```python
from build123d import *

# Parameters (mm, degrees)
F2_DEPTH = 18
F3_DEPTH = 188


with BuildPart() as f2:
    # F0 (on Front) → F2 (new body)
    with BuildSketch(Plane.XZ):
        with BuildLine():
            Line((63.480214, -200), (80, -200))
            ThreePointArc((80, -200), (94.142136, -194.142136), (100, -180))
            Line((100, -180), (100, 200))
            Line((100, 200), (45, 200))
            Line((45, 200), (45, 218))
            Line((45, 218), (-45, 218))
            Line((-45, 218), (-45, 200))
            Line((-45, 200), (-100, 200))
            Line((-100, 200), (-100, -180))
            ThreePointArc((-100, -180), (-94.142136, -194.142136), (-80, -200))
            Line((-80, -200), (-63.480214, -200))
            ThreePointArc((-63.480214, -200), (-49.338079, -194.142136), (-43.480214, -180))
            Line((-43.480214, -180), (-43.480214, -110))
            Line((-43.480214, -110), (-43.480214, 90))
            ThreePointArc((-43.480214, 90), (-37.62235, 104.142136), (-23.480214, 110))
            Line((-23.480214, 110), (23.480214, 110))
            ThreePointArc((23.480214, 110), (37.62235, 104.142136), (43.480214, 90))
            Line((43.480214, 90), (43.480214, -110))
            Line((43.480214, -110), (43.480214, -180))
            ThreePointArc((43.480214, -180), (49.338079, -194.142136), (63.480214, -200))
        make_face()
    extrude(amount=F2_DEPTH)

    # F1 (on face) → F3 (cut)
    with BuildSketch(Plane.XZ):
        Polygon((9, 170.049076), (-9, 170.049076), (-9, 110.049076), (0, 110.049076), (9, 110.049076), align=None)
        Polygon((0, 110.049076), (-9, 110.049076), (-9, 70.049076), (9, 70.049076), (9, 110.049076), align=None)
    extrude(amount=F3_DEPTH, mode=Mode.SUBTRACT)


solid = f2.part
```
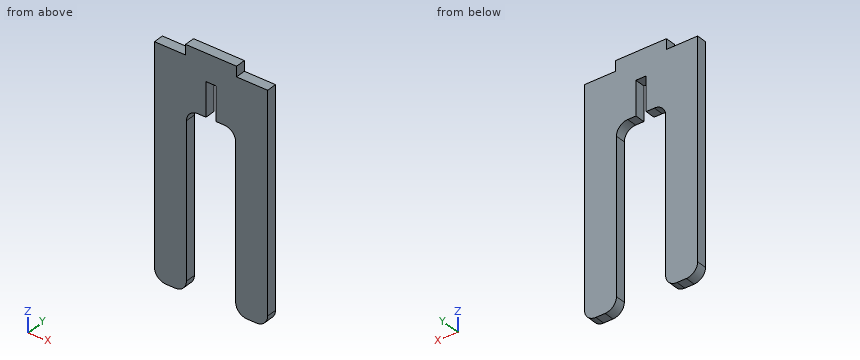
Read the model definition and answer for the solid it produces. Units are mm, in the model's axes. Round coordinates to 2 decimals unless told otherwise and drop trailing zeros. Write each loop counter-clockwise with the first axis right and the second up, starting at its lowest first coordinate (ties: lowest second). Pieces come first, ordered by that corner, then holes. Notation, with made-up numbers: (-17.75, 62.25) - (-2.75, 62.25) arc R10 ccw to (-2.75, 77.25) - close; hole circle Ø1 at (-17, -11). An arc over 180 degrees is marked (long way). One line per item, written item: value.
Q1. Each of these flat-tipped pins is pushed along its axis until it touches: P1, Ø9, axis at x = -59, y = -12.5, coming from the +Z side; P2, Ø7, axis at x = -18.5, y = -10, coming from the -Z side; P3, Ø4, axis at x = 57.5, y = -15.5, coming from the -Z side. Where does it stop, or does it pass through?
The answers:
P1: stops at z = 200
P2: stops at z = 110
P3: stops at z = -199.6
Q2. Find section C-C (z = 125). Determine the outline of the cut face in (x, y), and give its area (3 significant figures).
The answers:
outline: (-100, -18) - (-9, -18) - (-9, 0) - (-100, 0) - close; (9, -18) - (100, -18) - (100, 0) - (9, 0) - close
area: 3,280 mm2
Q3. Find section A-A (z = -117). Determine the outline of the cut face in (x, y).
The answers:
outline: (-100, -18) - (-43.48, -18) - (-43.48, 0) - (-100, 0) - close; (43.48, -18) - (100, -18) - (100, 0) - (43.48, 0) - close
Q4. Straight lines are drawn through the part: line 1 (X direction, y = -16.75, z = -69.5); line 2 (X direction, y = -2, z = 143.5); line 3 (Z direction, x = 11, y = -13.25). For each, find the intervals that lie inside material, in ascending order. Write a range as from..to.
The answers:
line 1: x = -100..-43.48, 43.48..100
line 2: x = -100..-9, 9..100
line 3: z = 110..218
Q5. Find section B-B (y = -11.5). Determine the outline of the cut face in (x, z), and give its area (3 significant figures).
The answers:
outline: (-100, -180) arc R20 ccw to (-80, -200) - (-63.48, -200) arc R20 ccw to (-43.48, -180) - (-43.48, 90) arc R20 cw to (-23.48, 110) - (-9, 110) - (-9, 170.05) - (9, 170.05) - (9, 110) - (23.48, 110) arc R20 cw to (43.48, 90) - (43.48, -180) arc R20 ccw to (63.48, -200) - (80, -200) arc R20 ccw to (100, -180) - (100, 200) - (45, 200) - (45, 218) - (-45, 218) - (-45, 200) - (-100, 200) - close
area: 53,400 mm2
Q6. Find section D-D (x = -16). Determine the outline of the cut face in (y, z), and give its area (3 significant figures).
The answers:
outline: (-18, 110) - (0, 110) - (0, 218) - (-18, 218) - close
area: 1,940 mm2
